from build123d import *

# Parameters (mm, degrees)
F1_DEPTH = 6.8
F2_R     = 4
F3_DEPTH = 25
F4_SIZE  = 1
F5_R     = 2


with BuildPart() as f1:
    # F0 (on Top) → F1 (new body)
    with BuildSketch(Plane.XY):
        Polygon((7.485782, 0.544427), (3.271403, 6.755091), (-4.214379, 6.210664), (-7.485782, -0.544427), (-3.271403, -6.755091), (4.214379, -6.210664), align=None)
    extrude(amount=F1_DEPTH)

    # F2 (on face) → F3 (join)
    with BuildSketch(Plane(origin=(0, 0, 0), x_dir=(1, 0, 0), z_dir=(0, 0, -1))):
        Circle(F2_R)
    extrude(amount=F3_DEPTH)

    # F4
    f4_edges = [f1.edges().sort_by_distance(p)[0] for p in [
        (-4, 0, -25),
    ]]
    chamfer(f4_edges, length=F4_SIZE)

    # F5
    f5_edges = [f1.edges().sort_by_distance(p)[0] for p in [
        (0.471488, -6.482877, 6.8),
        (-5.378592, -3.649759, 6.8),
        (-5.85008, 2.833118, 6.8),
        (-0.471488, 6.482877, 6.8),
        (5.378592, 3.649759, 6.8),
        (5.85008, -2.833118, 6.8),
        (7.485782, 0.544427, 3.4),
        (4.214379, -6.210664, 3.4),
        (-3.271403, -6.755091, 3.4),
        (-7.485782, -0.544427, 3.4),
        (-4.214379, 6.210664, 3.4),
        (3.271403, 6.755091, 3.4),
    ]]
    fillet(f5_edges, radius=F5_R)


solid = f1.part
Here's how the part is built. I have some questions about the finished solid (model axes, mm). A direction names the side the tool comes from. Coordinates: 2 decimals unless noted, no trailing zeros. Write each loop counter-clockwise with the first axis right and the second up, starting at its lowest first coordinate (ties: lowest second). Pieces come first, ordered by that corner, then holes.
Item 1: Will these pins go through, and if not, where does the flat tip stop? pin 1 (3 mm diameter, centred on y = 3.5, z = -15.5, fed in from -X); pin 2 (5 mm diameter, centred on y = 3, z = -2, fed in from +X); pin 3 (6 mm diameter, centred on x = -3.5, z = -18, fed in from -Y).
Item 2: I want a section at A-A on z = -20. Write out the boundary of the cut face in (x, y), and give its area (3 significant figures).
Item 3: On a 3-axis mill with a long thin cutter (end or side, diameter ignored), from which of +Z, -Z, +X, -X, +Y, -Y can I reach the whole of each face in a straight line? I mean faces 1 (the cylindrical face through (-4.03, 5.96, 2.43)), 2 (the flat face through (3, -3, 0)). Say none if no direction works.
Item 4: If I drill on line 1 (Z direction, x = 3.25, y = -3.5); line 2 (X direction, y = -0.5, z = 3.5); line 3 (Z direction, x = -4, y = -4.5), over which ranges is the centre line in solid material (lowest first)?
Findings below:
1. pin 1: stops at x = -3.46
1. pin 2: stops at x = 6.84
1. pin 3: stops at y = -3.97
2. outline: circle Ø8 at (0, 0)
2. area: 50.3 mm2
3. face 1: +Z, -Z, -X, +Y
3. face 2: -Z
4. line 1: z = 0 to 6.8
4. line 2: x = -7.18 to 6.98
4. line 3: z = 0 to 6.29
